Here's how the part is built. I have some questions about the finished solid (model axes, mm). Coordinates: 2 decimals unless noted, no trailing zeros. Write each loop counter-clockwise with the first axis right and the second up, starting at its lowest first coordinate (ties: lowest second). Pieces come first, ordered by that corner, then holes. Notation, with made-up numbers: (-9.75, -39.75) -> (29.25, -39.75) arc R22 cw to (29.25, -6.75) -> close; hole circle Ø8 at (-25.5, 28). An arc over 180 degrees is marked (long way). Put each result on its own line as item: value. Start each with the question number.
Item 1: For pin 1 (6.5 mm diameter, centred on x = 0, z = -12.7, fed in from -Y), with a flat end and sliding along its axis, tell me the tip position at first contact or that it passes through.
Item 2: I need wall thicknesses on line 1 (Z direction, x = 0.5, y = 0.1); line 2 (X direction, y = 1, z = 13); line 3 (X direction, y = 0.4, z = 12.7). Which ranges of each line are inside material? Lowest first, please. Write a range as [from, to].
Item 3: I want a section at B-B, the plane x = 1.5. State how many separate pieces and enclosed holes the cut face has, then the cut area to 3 significant figures.
Item 4: I want a section at A-A, the plane z = -12.7. List the corners of the cut face in (x, y) for me, then the cut area to 3 significant figures.
from build123d import *

# Parameters (mm, degrees)
SKETCH1_W      = 15.08125
SKETCH1_H      = 34.925
EXTRUDE1_DEPTH = 1.2
SKETCH3_R      = 2.1
EXTRUDE2_DEPTH = 1.984375
CHAMFER1_SIZE  = 0.508
FILLET1_R      = 7.540625
FILLET2_R      = 7.540625


with BuildPart() as part:
    # Sketch1 → Extrude1 (new body)
    with BuildSketch(Plane(origin=(0, 0, 0), x_dir=(1, 0, 0), z_dir=(0, 1, 0))):
        Rectangle(SKETCH1_W, SKETCH1_H)
    extrude(amount=EXTRUDE1_DEPTH)

    # Sketch3 → Extrude2 (cut)
    with BuildSketch(Plane(origin=(0, 1.2, 0), x_dir=(1, 0, 0), z_dir=(0, 1, 0))):
        with Locations(Location((0, 12.7, 0), (0, 0, 270))):
            Circle(SKETCH3_R)
        with Locations(Location((0, -12.7, 0), (0, 0, 270))):
            Circle(SKETCH3_R)
    extrude(amount=-EXTRUDE2_DEPTH, mode=Mode.SUBTRACT)

    # Chamfer1
    chamfer1_edges = [part.edges().sort_by_distance(p)[0] for p in [
        (0, 1.2, -14.8),
        (0, 1.2, 10.6),
    ]]
    chamfer(chamfer1_edges, length=CHAMFER1_SIZE)

    # Fillet1
    fillet1_edges = [part.edges().sort_by_distance(p)[0] for p in [
        (-7.540625, 0.6, -17.4625),
    ]]
    fillet(fillet1_edges, radius=FILLET1_R)

    # Fillet2
    fillet2_edges = [part.edges().sort_by_distance(p)[0] for p in [
        (7.540625, 0.6, 17.4625),
        (-7.540625, 0.6, 17.4625),
        (7.540625, 0.6, -17.4625),
    ]]
    fillet(fillet2_edges, radius=FILLET2_R - 0.0001)  # a hair under: the kernel refuses the full size


solid = part.part
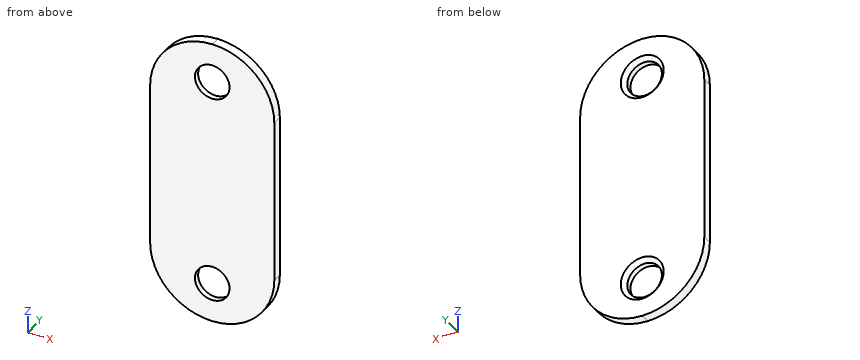
Calculated:
1. pin 1: stops at y = 0
2. line 1: z = [-17.45, -14.74], [-10.66, 10.66], [14.74, 17.45]
2. line 2: x = [-6.88, -2.39], [2.39, 6.88]
2. line 3: x = [-7.01, -2.1], [2.1, 7.01]
3. separate pieces: 3
3. enclosed holes: 0
3. area: 33.8 mm2
4. outline: (-7.01, 0) -> (-2.1, 0) -> (-2.1, 0.69) -> (-2.61, 1.2) -> (-7.01, 1.2) -> close; (2.1, 0) -> (7.01, 0) -> (7.01, 1.2) -> (2.61, 1.2) -> (2.1, 0.69) -> close
4. area: 11.5 mm2
